from build123d import *

# Parameters (mm, degrees)
BOSS_EXTRUDE1_DEPTH = 2.8
MIRROR1_START       = -2.8
MIRROR1_DEPTH       = 2.8
CHAMFER2_SIZE       = 0.2
BOSS_EXTRUDE2_DEPTH = 1
SKETCH2_W           = 18
SKETCH2_H           = 18
BOSS_EXTRUDE3_DEPTH = 5
BOSS_EXTRUDE3_TAPER = 10
FILLET1_R           = 1


# Read off the part's stored shape, not the designer's step: Mirror1
with BuildPart() as part:
    # Sketch1 → Boss-Extrude1 (new body)
    with BuildSketch(Plane(origin=(0, 0, 0), x_dir=(1, 0, 0), z_dir=(0, 1, 0))):
        Polygon((-2.85, 0), (-3.45, 0), (-3.45, 0.5), (-3.25, 0.7), (-3.25, 1.2), (-3.45, 1.4), (-3.45, 1.8), (-3.25, 2), (-2.85, 2), align=None)
    extrude(amount=-BOSS_EXTRUDE1_DEPTH)

    # Mirror1 outline → Mirror1 (add)
    with BuildSketch(Plane(origin=(0, 0, 0), x_dir=(1, 0, 0), z_dir=(0, 1, 0)).offset(MIRROR1_START)):
        Polygon((-2.85, 0), (-3.45, 0), (-3.45, -0.5), (-3.25, -0.7), (-3.25, -1.2), (-3.45, -1.4), (-3.45, -1.8), (-3.25, -2), (-2.45, -2), (-2.25, -1.8), (-2.25, -1.4), (-2.45, -1.2), (-2.45, -0.7), (-2.25, -0.5), (-2.25, 0.5), (-2.45, 0.7), (-2.45, 1.2), (-2.25, 1.4), (-2.25, 1.8), (-2.45, 2), (-2.85, 2), align=None)
    extrude(amount=MIRROR1_DEPTH)

    # Chamfer2
    chamfer2_edges = [part.edges().sort_by_distance(p)[0] for p in [
        (-2.85, -2.8, -2),
        (-3.35, -2.8, -1.9),
        (-3.45, -2.8, -1.6),
        (-3.35, -2.8, -1.3),
        (-3.25, -2.8, -0.95),
        (-2.35, -2.8, -0.6),
        (-2.25, -2.8, 0),
        (-2.35, -2.8, 0.6),
        (-2.85, -2.8, 2),
        (-3.35, -2.8, 1.9),
        (-3.45, -2.8, 1.6),
        (-3.35, -2.8, 1.3),
        (-3.25, -2.8, 0.95),
        (-2.35, -2.8, -1.9),
        (-2.25, -2.8, -1.6),
        (-2.35, -2.8, -1.3),
        (-2.45, -2.8, -0.95),
        (-3.35, -2.8, 0.6),
        (-3.35, -2.8, -0.6),
        (-2.45, -2.8, 0.95),
        (-2.35, -2.8, 1.3),
        (-2.25, -2.8, 1.6),
        (-2.35, -2.8, 1.9),
        (-3.45, -2.8, 0),
    ]]
    chamfer(chamfer2_edges, length=CHAMFER2_SIZE)


with BuildPart() as body_2:
    # Mirror5: mirrored copy
    add(part.part.mirror(Plane(origin=(0, 0, 0), x_dir=(0, 0, 1), z_dir=(1, 0, 0))))


with BuildPart() as part_1:
    add(part.part)

    add(body_2.part)  # Boss-Extrude2 merges body 2
    # Sketch1<4> → Boss-Extrude2 (add)
    # profile 1 of 2: a face of its own
    with BuildSketch(Plane(origin=(0, 0, 0), x_dir=(1, 0, 0), z_dir=(0, 1, 0))):
        Polygon((-5, 1.7), (-4.6, 2.1), (4.6, 2.1), (5, 1.7), (5, -1.7), (4.6, -2.1), (-4.6, -2.1), (-5, -1.7), align=None)
        Polygon((-2.85, 2), (-2.85, 0), (-3.45, 0), (-3.45, 0.5), (-3.25, 0.7), (-3.25, 1.2), (-3.45, 1.4), (-3.45, 1.8), (-3.25, 2), align=None, mode=Mode.SUBTRACT)
    # profile 2 of 2: a face of its own
    with BuildSketch(Plane(origin=(0, 0, 0), x_dir=(1, 0, 0), z_dir=(0, 1, 0))):
        Polygon((-2.85, 0), (-3.45, 0), (-3.45, 0.5), (-3.25, 0.7), (-3.25, 1.2), (-3.45, 1.4), (-3.45, 1.8), (-3.25, 2), (-2.85, 2), align=None)
    extrude(amount=BOSS_EXTRUDE2_DEPTH)

    # Sketch2 → Boss-Extrude3 (add)
    with BuildSketch(Plane(origin=(0, 0, 0), x_dir=(1, 0, 0), z_dir=(0, 1, 0))):
        Rectangle(SKETCH2_W, SKETCH2_H)
    extrude(amount=BOSS_EXTRUDE3_DEPTH, taper=BOSS_EXTRUDE3_TAPER)

    # Fillet1
    fillet1_edges = [part_1.edges().sort_by_distance(p)[0] for p in [
        (8.559182548, 2.5, 8.559182548),
        (8.559182548, 2.5, -8.559182548),
        (-8.559182548, 2.5, -8.559182548),
        (-8.559182548, 2.5, 8.559182548),
    ]]
    fillet(fillet1_edges, radius=FILLET1_R)


solid = part_1.part
CAD build for the part. Positions are in the model's coordinates, mm. A direction names the side the tool comes from. Round coordinates to 2 decimals unless told otherwise and drop trailing zeros. Use a Markdown table: item, result. Add a question column.
1. 3-axis set-ups, long thin cutter, end or side, ignore diameter. For faces 1 (the face through (-2.25, -1, 0)), 2 (the face through (-3.45, -1, 0)), 3 (the face through (-3, -2.8, 0)): which of +Z, -Z, +X, -X, +Y, -Y reach the whole face in a straight line?
2. Flat gauge pins, fed straight in: P1, Ø0.6, axis at x = -3, y = -1.5, coming from the +Z side; P2, Ø0.6, axis at x = -3, y = -0.5, coming from the -Z side; P3, Ø2, axis at x = -3.5, y = 3.5, coming from the -Z side. Where does each tip first touch, or does it go through?
3. Pull direction X, two halves, no side cores. Call faces 4 (the face through (3, -2.8, 0)), 5 (the face through (2.25, -1, 0)), 6 (the face through (3.45, -1, 0)): released by +X, released by -X, zero draft, split by the parting line, or undercut.
4. Drill centre lines: probe 1 along Y at (x, z) = (-1.5, 5.5); probe 2 along Z at (x, y) = (-3, 0.25); probe 3 along X at (y, z) = (2.5, 7). Where is each one in solid material? Low to high.
Reply:
| question | item | result |
|---|---|---|
| 1 | face 1 | +Z, -Z, -Y |
| 1 | face 2 | +Z, -Z, -X, -Y |
| 1 | face 3 | +Z, -Z, +X, -X, -Y |
| 2 | P1 | stops at z = 2 |
| 2 | P2 | stops at z = -2 |
| 2 | P3 | stops at z = -8.56 |
| 3 | face 4 | zero draft |
| 3 | face 5 | undercut |
| 3 | face 6 | released by +X |
| 4 | probe 1 | y = 0 to 5 |
| 4 | probe 2 | z = -8.96 to 8.96 |
| 4 | probe 3 | x = -8.56 to 8.56 |
